Autodesk Inventor part; units mm, degrees
ref_plane "YZ Plane" through (0, 0, 0) normal (1, 0, 0) x (0, 1, 0)
ref_plane "XZ Plane" through (0, 0, 0) normal (0, 1, 0) x (-1, 0, 0)
ref_plane "XY Plane" through (0, 0, 0) normal (0, 0, 1) x (1, 0, 0)
sketch "Sketch1" plane through (0, 0, 0) normal (1, 0, 0) x (0, 1, 0)
  line L0 (0, 0) -> (0, 30)
  line L1 (0, 30) -> (20, 30)
  line L2 (20, 30) -> (20, -60)
  line L3 (20, -60) -> (0, -60)
  line L4 (0, -60) -> (0, 30)
  line L5 (20, 30) -> (30, 30)
  line L6 (30, 30) -> (30, -30)
  line L7 (30, -30) -> (20, -30)
  line L8 (20, -30) -> (20, 30)
  line L9 (0, 30) -> (20, 30)
  line L10 (20, 30) -> (20, 45)
  line L11 (20, 45) -> (0, 45)
  line L12 (0, 45) -> (0, 30)
  line L13 (20, 0) -> (0, 0)
  line L14 (0, -60) -> (20, -30)
  line L15 (20, -30) -> (30, -30)
  line L16 (0, -60) -> (20, -30)
  line L17 (20, -30) -> (20, -45)
  line L18 (20, -45) -> (0, -45)
  line L19 (0, -45) -> (0, -60)
  line L20 (20, 45) -> (30, 30)
  line L21 (30, -30) -> (20, -45)
  line L22 (20, -30) -> (0, -30)
  point P0 (20, -30)
  point P1 (20, -30)
  point P2 (20, -30)
  point P3 (10, -45)
  point P4 (20, -30)
  point P5 (0, -45)
  point P6 (10, -45)
  dimension "d0" = 30
  dimension "d1" = 20
  dimension "d2" = 90
  dimension "d3" = 10
  dimension "d4" = 20
  dimension "d5" = 15
extrude "Extrusion1" add sketch "Sketch1" along normal blind 20 contours L12 L11 L10 L1 | L22 L14 L18 L4 | L2 L5 L6 L7 | L10 L20 L5 | L7 L21 L2 | L2 L18 L14
fillet "Fillet2" radius 45.25 2 edges at (10, 30, -30) (10, 30, 30)
fillet "Fillet3" radius 11 2 edges at (10, 20, 30) (10, 20, -30)
fillet "Fillet4" radius 22.25 2 edges at (10, 20, -45) (10, 20, 45)
sketch "Sketch3" plane through (0, 0, -45) normal (0, -1, 0) x (1, 0, 0)
  circle A0 centre (14, 7.5) radius 3.25
  line L0 (0, 0) -> (20, 0)
  circle A1 centre (6, 7.5) radius 1
  line L1 (0, 45) -> (21.3664, 45)
  circle A2 centre (14, 82.5) radius 3.25
  circle A3 centre (6, 82.5) radius 1
  line L2 (20, 15) -> (20, 0)
  line L3 (0, 15) -> (0, 0)
  point P0 (20, 90)
  point P1 (20, 7.5)
  dimension "d21" = 6.5
  dimension "d22" = 7.5
  dimension "d23" = 2
  dimension "d28" = 7.5
  dimension "d29" = 6
  dimension "d30" = 6
extrude "Extrusion4" cut sketch "Sketch3" against normal blind 3.5 contours A0 | A2
extrude "Extrusion5" cut sketch "Sketch3" against normal blind 10 contours A1 | A3
properties part number "Raczka"
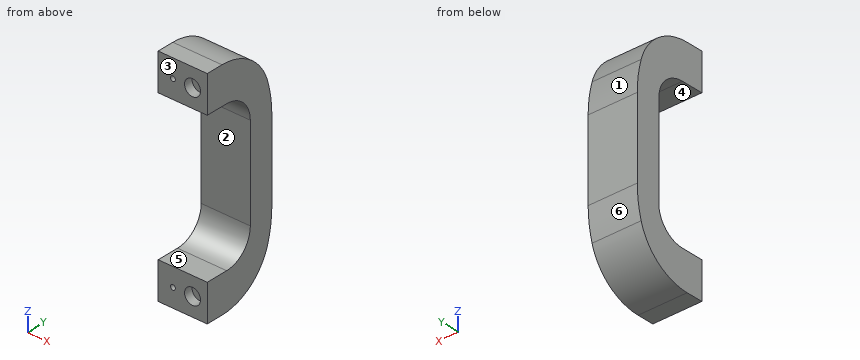
The model under review builds one solid part; all positions refer to its coordinate system, in mm. Face numbers are marked on the shaded views. A direction names the side the tool comes from. Coordinates: 2 decimals unless noted, no trailing zeros. Write each loop counter-clockwise with the first axis right and the second up, starting at its lowest first coordinate (ties: lowest second). Pieces come first, ordered by that corner, then holes. Notation, with made-up numbers: (80, 1.25) - (106, 1.25) arc R13 ccw to (106, 12.25) - close; hole circle Ø5 at (57, 76). An arc over 180 degrees is marked (long way). Answer in a Markdown table with one row per item. Add a question column.
Q1. Consider section B-B on z = -6.5. Give the boundary of the cut face in (x, y).
Q2. For the marked faces 1 and 2, list the 3-axis set-ups (+Z, -Z, +X, -X, +Y, -Y) from which the entire face can be reached by the end or side of a thin tool; tool diameter is ignored.
Q3. Clearance check with flat-ended pins moving along their axes: pin 1 (2 mm diameter, centred on x = 9, z = 19.5, fed in from -Y); pin 2 (8 mm diameter, centred on y = 20, z = 12, fed in from -X); pin 3 (1.2 mm diameter, centred on x = 6, z = -37.5, fed in from +Y); pin 4 (5 mm diameter, centred on x = 14, z = 37, fed in from -Y). State where each tip first meets the part, or that it passes through.
Q4. Draft analysis for pull direction Z (two halves, no side actions). For the marked faces 3, 4, 5 and 6, state which applies: +Z half, -Z half, draft (parallel to the pull), parting line (faces both ways), or undercut.
Q5. To check wall thickness, follow line 1 along Z through (x, y) = (6, 2.5); line 2 along Z through (x, y) = (14, 1.45); line 3 along Z through (x, y) = (11.25, 6). State the ranges of each line that lie inside material, in increasing order. Write a range as from..to.
Q6. Consider section A-A on y = 6. Give the boundary of the cut face in (x, z), then the cut area to 3 significant figures.
Answers below:
| question | item | result |
|---|---|---|
| 1 | outline | (0, 20) - (20, 20) - (20, 30) - (0, 30) - close |
| 2 | face 1 | +Z, +X, -X, +Y |
| 2 | face 2 | +X, -X, -Y |
| 3 | pin 1 | y = 19.9 |
| 3 | pin 2 | x = 0 |
| 3 | pin 3 | y = 24 |
| 3 | pin 4 | y = 3.5 |
| 4 | face 3 | draft |
| 4 | face 4 | undercut |
| 4 | face 5 | undercut |
| 4 | face 6 | -Z half |
| 5 | line 1 | -45..-38.5, -36.5..-30, 30..36.5, 38.5..45 |
| 5 | line 2 | -45..-40.75, -34.25..-30, 30..34.25, 40.75..45 |
| 5 | line 3 | -45..-30, 30..45 |
| 6 | outline | (0, -45) - (20, -45) - (20, -30) - (0, -30) - close; (0, 30) - (20, 30) - (20, 45) - (0, 45) - close; hole circle Ø2 at (6, -37.5); hole circle Ø2 at (6, 37.5) |
| 6 | area | 594 mm² |
